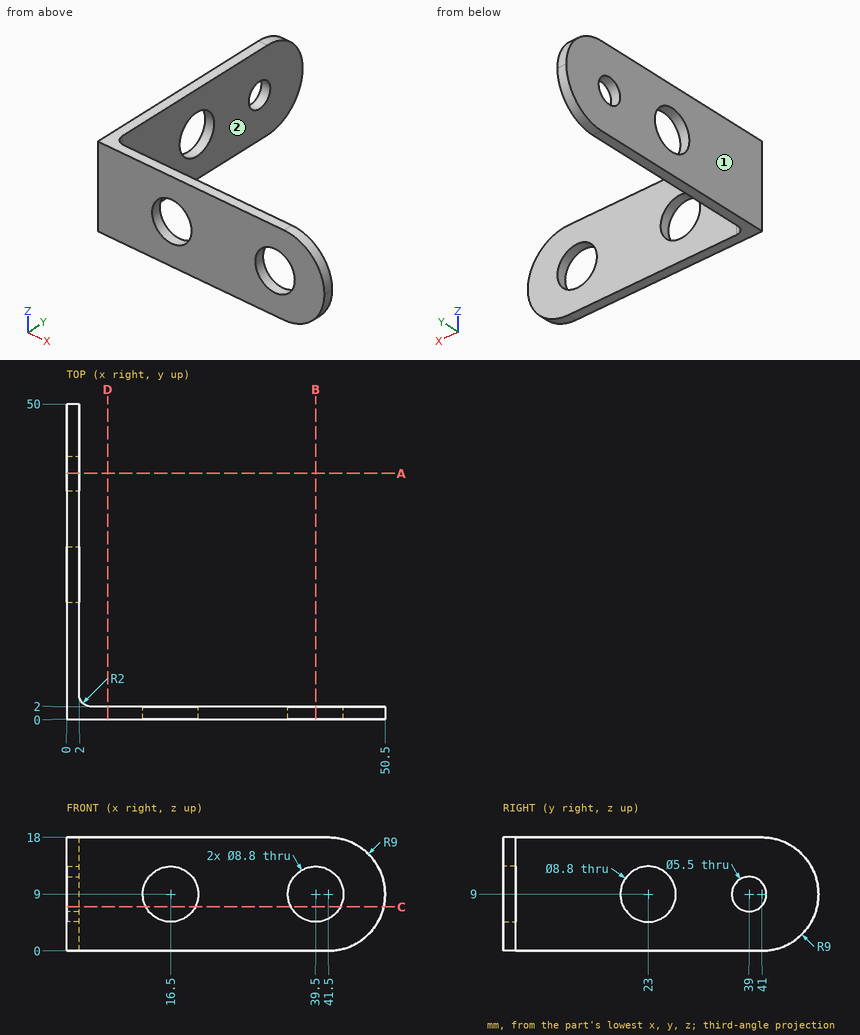
Design review of the part shown in the three views and the two pictorial views. Dimensions are in mm from the part's minimum x, y and z. A direction names the side the tool comes from. Round coordinates to 2 decimals unless told otherwise and drop trailing zeros. Order: outer loops, then holes, each group sorted by start corner. A loop starts at its lowest first (then second) coordinate and runs counter-clockwise, first axis right, second up. Notation, with made-up numbers: (43, -9.75) -> (68, -9.75) arc R36 cw to (68, 24.25) -> close; hole circle Ø10 at (76.25, 82). An arc over 180 degrees is marked (long way). Write item = value, one per line. Start each with the question number.
1) Take a section at A-A on y = 39. State the section outline as (x, z) points.
2) Take a section at D-D on x = 6.5. State the section outline as (y, z) points, plus the area to 3 significant figures.
3) Tool access review of the marked faces 1 and 2: name each direction out of +Z, -Z, +X, -X, +Y, -Y from which nothing blocks a thin tool from reaching the whole face with its end or side.
4) Take a section at B-B on x = 39.5. State the section outline as (y, z) points, plus the area to 3 significant figures.
5) To check wall thickness, follow line 1 (X direction, y = 31, z = 4.5); line 2 (X direction, y = 2.5, z = 8.75). State the ranges of each line that lie inside material, in increasing order. Write a range as from..to.
6) Insertion check: pin 1 (5.5 mm diameter, centred on y = 37.5, z = 13, fed in from +X); pin 2 (5.5 mm diameter, centred on x = 21, z = 13, fed in from +Y). Each pin has a flat end and moves straight along its axis. Give the tip position at first contact, or say it passes through.
7) Take a section at C-C on z = 7. State the section outline as (x, y) points, plus the area to 3 significant figures.
Verdict:
q1.outline = (0, 0) -> (2, 0) -> (2, 6.25) -> (0, 6.25) -> close; (0, 11.75) -> (2, 11.75) -> (2, 18) -> (0, 18) -> close
q2.outline = (0, 0) -> (2, 0) -> (2, 18) -> (0, 18) -> close
q2.area = 36.0 mm2
q3.face_1 = +Z, -Z, -X, +Y, -Y
q3.face_2 = +Z, -Z, +X, +Y
q4.outline = (0, 0) -> (2, 0) -> (2, 4.6) -> (0, 4.6) -> close; (0, 13.4) -> (2, 13.4) -> (2, 18) -> (0, 18) -> close
q4.area = 18.4 mm2
q5.line_1 = 0..2
q5.line_2 = 0..2.68
q6.pin_1 = 2
q6.pin_2 = 2
q7.outline = (0, 0) -> (12.58, 0) -> (12.58, 2) -> (4, 2) arc R2 cw to (2, 4) -> (2, 19.08) -> (0, 19.08) -> close; (0, 26.92) -> (2, 26.92) -> (2, 37.11) -> (0, 37.11) -> close; (0, 40.89) -> (2, 40.89) -> (2, 49.77) -> (0, 49.77) -> close; (20.42, 0) -> (35.58, 0) -> (35.58, 2) -> (20.42, 2) -> close; (43.42, 0) -> (50.27, 0) -> (50.27, 2) -> (43.42, 2) -> close
q7.area = 142 mm2
